Input: part model. Units: mm. Frame: model coordinates. A direction names the side the tool comes from. Round coordinates to 2 decimals unless told otherwise and drop trailing zeros. Order: outer loops, then holes, each group sorted by start corner. A loop starts at its lowest first (then second) coordinate and runs counter-clockwise, first axis right, second up. Notation, with made-up numbers: M -26,-30 L -17,-30 A23 ccw -17,4 Z; hole C 87.25,-37.5 d11. An arc over 180 degrees is marked long. One line per question, with ' | ' between items.
```python
from build123d import *

# Parameters (mm, degrees)
SKETCH1_W      = 60
SKETCH1_H      = 30
SKETCH1_R      = 3.5
EXTRUDE1_DEPTH = 15
EXTRUDE2_DEPTH = 7.5
EXTRUDE3_DEPTH = 31
FILLET1_R      = 0.5


with BuildPart() as part:
    # Sketch1 → Extrude1 (new body)
    with BuildSketch(Plane.XY):
        with Locations((0, -15)):
            Rectangle(SKETCH1_W, SKETCH1_H)
        with Locations((20, -10)):
            Circle(SKETCH1_R, mode=Mode.SUBTRACT)
        with Locations((-20, -10)):
            Circle(SKETCH1_R, mode=Mode.SUBTRACT)
    extrude(amount=-EXTRUDE1_DEPTH)

    # Sketch2 → Extrude2 (cut)
    with BuildSketch(Plane.XY):
        with BuildLine():
            Line((13, -20), (30, -20))
            Line((30, -20), (30, 0))
            Line((30, 0), (10, 0))
            Line((10, 0), (10, -17))
            ThreePointArc((10, -17), (10.878679656, -19.121320344), (13, -20))
        make_face()
        with BuildLine():
            Line((-30, -20), (-30, 0))
            Line((-30, 0), (-10, 0))
            Line((-10, 0), (-10, -17))
            ThreePointArc((-10, -17), (-10.878679656, -19.121320344), (-13, -20))
            Line((-13, -20), (-30, -20))
        make_face()
    extrude(amount=-EXTRUDE2_DEPTH, mode=Mode.SUBTRACT)

    # Sketch3 → Extrude3 (cut, through all)
    with BuildSketch(Plane(origin=(0, 0, 0), x_dir=(1, 0, 0), z_dir=(0, 1, 0))):
        with BuildLine():
            Line((6, 0), (6, 5))
            ThreePointArc((6, 5), (0, 11), (-6, 5))
            Line((-6, 5), (-6, 0))
            Line((-6, 0), (6, 0))
        make_face()
    extrude(amount=-EXTRUDE3_DEPTH, mode=Mode.SUBTRACT)

    # Fillet1
    fillet1_edges = [part.edges().sort_by_distance(p)[0] for p in [
        (21.5, -20, -7.5),
        (10.878679656, -19.121320344, -7.5),
        (10, -8.5, -7.5),
        (-10.878679656, -19.121320344, -7.5),
        (-21.5, -20, -7.5),
        (-10, -8.5, -7.5),
    ]]
    fillet(fillet1_edges, radius=FILLET1_R)


solid = part.part
```
Item 1: First-contact query: pin 1 (1.5 mm diameter, centred on x = 1.5, z = -13.5, fed in from +Y); pin 2 (5.5 mm diameter, centred on x = 20, y = -10, fed in from -Z); pin 3 (2 mm diameter, centred on y = -12, z = -2, fed in from -X); pin 4 (5.5 mm diameter, centred on y = -15, z = -3, fed in from +X). Flat tips, straight axial feed; report the tip coordinate or a pass-through.
Report:
pin 1: y = 0 | pin 2: through | pin 3: x = -10 | pin 4: x = 10.1
Item 2: Mould query, pull axis Y, two halves, no side actions, for faces 6 (the flat face through (-6, -15, -3)), 7 (the cylindrical face through (-16.767, -11.341, -11.198)), 8 (the flat face through (-21, -20, -3)). Classes: +Y half, -Y half, draft (parallel to the pull), parting line (faces both ways), or undercut.
Report:
face 6: draft | face 7: undercut | face 8: +Y half
Item 3: Section query C-C, the plane z = -8.25. Return loops of the section in (x, y).
Report:
outline: M -30,-30 L -5.04,-30 L -5.04,0 L -30,0 Z; M 5.04,-30 L 30,-30 L 30,0 L 5.04,0 Z; hole C -20,-10 d7; hole C 20,-10 d7
Item 4: Access query for faces 1 (the flat face through (0, -15, -15)), 2 (the cylindrical face through (10.86, -19.1, -3.45)), 3 (the flat face through (15, -21, 0)), 4 (the flat face through (6, -15, -2)), 5 (the flat face through (-10, -8, -3)). Directions: +Z, -Z, +X, -X, +Y, -Y. A direction counts if a zero-diameter tool reaches every point of the face in a straight line with its end or side. Return the directions, or none.
Report:
face 1: -Z, +X, -X, +Y, -Y | face 2: +Z, +X, +Y | face 3: +Z, +X, -X, +Y, -Y | face 4: +Z, +Y, -Y | face 5: +Z, -X, +Y
Item 5: Section query D-D, the plane y = -27.5. Return loops of the section in (x, z).
Report:
outline: M -30,-15 L 30,-15 L 30,0 L 6,0 L 6,-5 A6 cw -6,-5 L -6,0 L -30,0 Z
Item 6: Section query A-A, the plane x = 20. Return loops of the section in (y, z).
Report:
outline: M -30,-15 L -13.5,-15 L -13.5,-7.5 L -19.5,-7.5 A0.5 cw -20,-7 L -20,0 L -30,0 Z; M -6.5,-15 L 0,-15 L 0,-7.5 L -6.5,-7.5 Z
Item 7: Line query: line 1 along Y through (x, z) = (20, -13); line 2 along X through (y, z) = (-15.25, -5.25); line 3 along X through (y, z) = (-22.75, -2.5). Output: solid intervals per line, ascending. Write a range as from..to.
Report:
line 1: -30..-13.5, -6.5..0 | line 2: -10..-5.99, 5.99..10 | line 3: -30..-6, 6..30
Item 8: Section query B-B, the plane y = -10. Return loops of the section in (x, z), plus the area to 3 significant figures.
Report:
outline: M -30,-15 L -23.5,-15 L -23.5,-7.5 L -30,-7.5 Z; M -16.5,-15 L 16.5,-15 L 16.5,-7.5 L 10.5,-7.5 A0.5 cw 10,-7 L 10,0 L 6,0 L 6,-5 A6 cw -6,-5 L -6,0 L -10,0 L -10,-7 A0.5 cw -10.5,-7.5 L -16.5,-7.5 Z; M 23.5,-15 L 30,-15 L 30,-7.5 L 23.5,-7.5 Z | area: 379 mm²
